The listing builds one solid part. Answer for the finished solid, in the listing's coordinates (mm). A direction names the side the tool comes from. Round coordinates to 2 decimals unless told otherwise and drop trailing zeros. Loops run counter-clockwise (first coordinate to the right, second up) from the corner with the lowest first, then second, coordinate; pieces in that order, holes last. Notation, with made-up numbers: (20, 4) - (52, 4) arc R32 cw to (52, 30) - close; hole circle Ø5 at (35, 9.25). An arc over 180 degrees is marked (long way). One line per question, with ' | ' between items. Start each with the question number.
from build123d import *

# Parameters (mm, degrees)
F0_R      = 12.7
F1_DEPTH  = 60.325
F2_R      = 5.08
F3_R      = 7.874
F5_DEPTH  = 19.05
F7_DEPTH  = 41.275
F8_R      = 6.35
F9_DEPTH  = 22.951227039
F10_R     = 5.08
F11_R     = 5.08
F13_W     = 63.8135012672
F13_H     = 22.225
F14_DEPTH = 57.15


with BuildPart() as f1:
    # F0 (on Top) → F1 (new body)
    with BuildSketch(Plane.XY):
        with BuildLine():
            ThreePointArc((-113.8312659101, -44.9580233222), (-153.8868240783, -31.9212818085), (-131.0386, -67.3100233222))
            Line((-131.0386, -67.3100233222), (-44.3288590271, -67.3100233222))
            Line((-44.3288590271, -67.3100233222), (-50.3232590271, -44.9580233222))
            Line((-50.3232590271, -44.9580233222), (-113.8312659101, -44.9580233222))
        make_face()
        with Locations((-136.1752590271, -45.5562503612)):
            Circle(F0_R, mode=Mode.SUBTRACT)
        Polygon((-50.3232590271, -44.9580233222), (-44.3288590271, -67.3100233222), (-18.9288590271, -67.3100233222), (-18.9288590271, -44.9580233222), align=None)
        Polygon((-18.9288590271, -44.9580233222), (-18.9288590271, -67.3100233222), (58.0331409729, -67.3100233222), (58.0331409729, -44.9580233222), (13.9133409729, -44.9580233222), align=None)
        with BuildLine():
            ThreePointArc((-5.1366590271, -10.1600233222), (-8.7108436655, -28.8756656882), (-18.9288590271, -44.9580233222))
            Line((-18.9288590271, -44.9580233222), (13.9133409729, -44.9580233222))
            Line((13.9133409729, -44.9580233222), (13.9133409729, -10.1600233222))
            Line((13.9133409729, -10.1600233222), (-5.1366590271, -10.1600233222))
        make_face()
    extrude(amount=F1_DEPTH)

    # F2
    f2_edges = [f1.edges().sort_by_distance(p)[0] for p in [
        (13.913341, -10.160023, 30.1625),
    ]]
    fillet(f2_edges, radius=F2_R)

    # F3
    f3_edges = [f1.edges().sort_by_distance(p)[0] for p in [
        (58.033141, -44.958023, 30.1625),
    ]]
    fillet(f3_edges, radius=F3_R)

    # F4 (on face) → F5 (cut)
    with BuildSketch(Plane.XY.offset(60.325)):
        Polygon((-18.9288590271, -67.3100233222), (-18.9288590271, -44.9580233222), (-50.3232590271, -44.9580233222), (-44.3288590271, -67.3100233222), align=None)
    extrude(amount=-F5_DEPTH, mode=Mode.SUBTRACT)

    # F6 (on face) → F7 (cut)
    with BuildSketch(Plane(origin=(0, 0, 0), x_dir=(1, 0, 0), z_dir=(0, 0, -1))):
        with BuildLine():
            Line((13.9133409729, 15.2400233222), (13.9133409729, 44.9580233222))
            Line((13.9133409729, 44.9580233222), (-18.9288590271, 44.9580233222))
            ThreePointArc((-18.9288590271, 44.9580233222), (-8.7108436655, 28.8756656882), (-5.1366590271, 10.1600233222))
            Line((-5.1366590271, 10.1600233222), (8.8333409729, 10.1600233222))
            ThreePointArc((8.8333409729, 10.1600233222), (12.4254434213, 11.6479208738), (13.9133409729, 15.2400233222))
        make_face()
    extrude(amount=-F7_DEPTH, mode=Mode.SUBTRACT)

    # F8 (on face) → F9 (cut, through all)
    with BuildSketch(Plane(origin=(0, -44.9580233222, 0), x_dir=(-1, 0, 0), z_dir=(0, 1, 0))):
        with Locations((-11.2971409729, 22.352)):
            Circle(F8_R)
    extrude(amount=-F9_DEPTH, mode=Mode.SUBTRACT)

    # F10
    f10_edges = [f1.edges().sort_by_distance(p)[0] for p in [
        (13.913341, -44.958023, 50.8),
    ]]
    fillet(f10_edges, radius=F10_R)

    # F11
    f11_edges = [f1.edges().sort_by_distance(p)[0] for p in [
        (-113.831266, -44.958023, 30.1625),
    ]]
    fillet(f11_edges, radius=F11_R)

    # F13 (on offset) → F14 (cut)
    with BuildSketch(Plane.YZ.offset(-160.02)):
        with Locations((-45.4811556265, 30.1625)):
            Rectangle(F13_W, F13_H)
    extrude(amount=F14_DEPTH, mode=Mode.SUBTRACT)


solid = f1.part
(1) A tool of negligible diameter and unlimited length cuts with its end or side. For faces 5 (the flat face through (-28, -44.958, 23)), 6 (the cylindrical face through (-112.498, -43.855, 50.933)), 7 (the flat face through (-125, -56, 19.05)), from which of +Z, -Z, +X, -X, +Y, -Y can it reach the whole face along a straight path? Write none if from no direction.
(2) Find section D-D on x = -57. Write down the section's boundary in (y, z) (3 decimals).
(3) Find section B-B on z = 9. Write down the section's boundary in (x, y).
(4) Consider L1, parallel to Z at x = -128, y = -63 (3 decimals); L2, parallel to X at y = -54, z = 54.5; L3, parallel to X at y = -35.5, z = 6.5. Determine where each line is inside the solid, lowest interval first.
(5) Find section A-A on y = -29.5. Write down the section's boundary in (x, z) (3 decimals), plus the area to 3 significant figures.
(6) Determine the mould class of faces 1 (the cylindrical face through (-124.444, -50.42, 50.667)), 2 (the flat face through (-102.87, -56, 30)), 3 (the cylindrical face through (55.665, -47.203, 30.585)), 4 (the flat face through (-38, -67.31, 30)) for opening direction Y: pulls with the +Y half, pulls with the -Y half, needs draft (parallel to the pull), parting line crosses it, or undercut.
(7) Find section C-C on x = -14. Write down the section's boundary in (y, z) (3 decimals), plus the area to 3 significant figures.
(8) Each of these flat-tipped pins is pushed along its axis until it touches: P1, Ø2, axis at y = -53.5, z = 28.5, coming from the -X side; P2, Ø5, axis at y = -26, z = 24, coming from the +X side; P3, Ø24.5, axis at x = -35.5, y = -57.5, coming from the +Z side (3 decimals); P4, Ø14.5, axis at x = 11.3, z = 22.35, coming from the -Y side. Where does it stop, or does it pass through?
Answer below:
1) face 5: -Z, +Y | face 6: +Z, -Z, +Y | face 7: -X, +Y, -Y
2) outline: (-67.31, 0) - (-44.958, 0) - (-44.958, 60.325) - (-67.31, 60.325) - close
3) outline: (-131.04, -67.31) - (58.03, -67.31) - (58.03, -52.83) arc R7.87 ccw to (50.16, -44.96) - (-109.34, -44.96) arc R5.08 cw to (-114.31, -40.93) arc R22.35 ccw (long way) to start; hole circle Ø25.4 at (-136.18, -45.56)
4) L1: 0 to 19.05, 41.275 to 60.325 | L2: -156.87 to -145.66, -126.69 to -47.9, -18.93 to 58.03 | L3: -156.14 to -143.93, -128.42 to -116.21
5) outline: (-151.725, 0) - (-120.625, 0) - (-120.625, 19.05) - (-151.725, 19.05) - close; (-151.725, 41.275) - (-120.625, 41.275) - (-120.625, 60.325) - (-151.725, 60.325) - close; (-8.963, 41.275) - (13.913, 41.275) - (13.913, 60.325) - (-8.963, 60.325) - close | area: 1,620 mm2
6) face 1: undercut | face 2: needs draft | face 3: pulls with the +Y half | face 4: pulls with the -Y half
7) outline: (-67.31, 0) - (-44.958, 0) - (-44.958, 41.275) - (-38.827, 41.275) - (-38.827, 60.325) - (-67.31, 60.325) - close | area: 1,470 mm2
8) P1: x = -102.87 | P2: through | P3: z = 60.325 | P4: y = -67.31
